Can you work these out from the drawing? Everything is in mm from the part's minimum corner. A direction names the side the tool comes from. Coordinates: 2 decimals unless noted, no trailing zeros. Order: outer loops, then holes, each group sorted by start corner. A loop starts at its lowest first (then second) coordinate and runs counter-clockwise, first axis right, second up. Notation, with made-up numbers: (-16.75, -40) - (-9.75, -40) arc R11 ccw to (-9.75, -28) - close; hole circle Ø7 at (40, 41.25). An arc over 180 degrees is marked (long way). Use a Markdown table: item, result. Add a question column.
(1) For pin 1 Ø3 at (x, y) = (41.5, 3.5) entering from +Z; pin 2 Ø1 at (x, z) = (10.5, 9) entering from -Y; pin 3 Ø6 at (x, z) = (30, 9) entering from +Y; pin 4 Ø1.5 at (y, z) = (2.5, 7) entering from -X, each with a flat end and sliding along its axis, tell me the tip position at first contact or that it passes through.
(2) On a 3-axis mill with a long thin cutter (end or side, diameter ignored), from which of +Z, -Z, +X, -X, +Y, -Y can I reach the whole of each face in a straight line? I mean the marked faces 4 and 5. Say none if no direction works.
(3) We'd pull the mould along Y, two halves only. Please class the marked faces 1, 2 and 3: pulls with the +Y half, pulls with the -Y half, needs draft (parallel to the pull), parting line crosses it, or undercut.
(4) I want a section at D-D (z = 8.25). List the corners of the cut face in (x, y) for me.
(5) I want a section at B-B (x = 22.5). List the corners of the cut face in (y, z) for me, and give its area (3 significant figures).
(6) I want a section at A-A (z = 6). List the corners of the cut face in (x, y) for me, and give its area (3 significant figures).
(7) I want a section at C-C (y = 4.5). List the corners of the cut face in (x, z) for me.
(8) If I drill on L1, parallel to X at y = 5.5, z = 1.5; L2, parallel to Z at x = 16.5, y = 3.4; L3, parallel to X at y = 5.75, z = 3, over which ranges is the centre line in solid material (lowest first)? Write a range as [from, to].
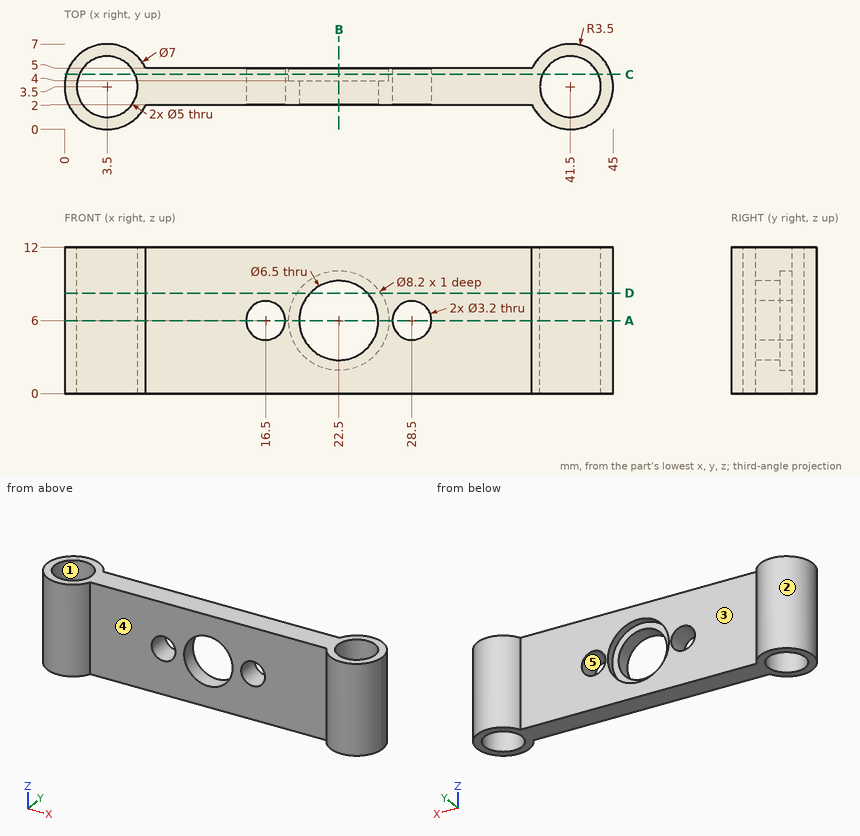
Answers follow:
| question | item | result |
|---|---|---|
| 1 | pin 1 | passes through |
| 1 | pin 2 | stops at y = 2 |
| 1 | pin 3 | stops at y = 5 |
| 1 | pin 4 | stops at x = 0.01 |
| 2 | face 4 | +Z, -Z, -Y |
| 2 | face 5 | +Y, -Y |
| 3 | face 1 | undercut |
| 3 | face 2 | parting line crosses it |
| 3 | face 3 | pulls with the +Y half |
| 4 | outline | (6.66, 2) - (20.15, 2) - (20.15, 4) - (19.07, 4) - (19.07, 5) - (6.66, 5) arc R3.5 ccw (long way) to start; (24.85, 2) - (38.34, 2) arc R3.5 ccw (long way) to (38.34, 5) - (25.93, 5) - (25.93, 4) - (24.85, 4) - close; hole circle Ø5 at (3.5, 3.5); hole circle Ø5 at (41.5, 3.5) |
| 5 | outline | (2, 0) - (5, 0) - (5, 1.9) - (4, 1.9) - (4, 2.75) - (2, 2.75) - close; (2, 9.25) - (4, 9.25) - (4, 10.1) - (5, 10.1) - (5, 12) - (2, 12) - close |
| 5 | area | 14.8 mm² |
| 6 | outline | (6.66, 2) - (14.9, 2) - (14.9, 5) - (6.66, 5) arc R3.5 ccw (long way) to start; (18.1, 2) - (19.25, 2) - (19.25, 4) - (18.4, 4) - (18.4, 5) - (18.1, 5) - close; (25.75, 2) - (26.9, 2) - (26.9, 5) - (26.6, 5) - (26.6, 4) - (25.75, 4) - close; (30.1, 2) - (38.34, 2) arc R3.5 ccw (long way) to (38.34, 5) - (30.1, 5) - close; hole circle Ø5 at (3.5, 3.5); hole circle Ø5 at (41.5, 3.5) |
| 6 | area | 91.0 mm² |
| 7 | outline | (0.15, 0) - (1.21, 0) - (1.21, 12) - (0.15, 12) - close; (5.79, 0) - (39.21, 0) - (39.21, 12) - (5.79, 12) - close; (43.79, 0) - (44.85, 0) - (44.85, 12) - (43.79, 12) - close; hole circle Ø3.2 at (16.5, 6); hole circle Ø8.2 at (22.5, 6); hole circle Ø3.2 at (28.5, 6) |
| 8 | L1 | x = [0.63, 2], [5, 6.37], [38.63, 40], [43, 44.37] |
| 8 | L2 | z = [0, 4.4], [7.6, 12] |
| 8 | L3 | x = [0.82, 2.41], [4.59, 6.18], [38.82, 40.41], [42.59, 44.18] |
